Work out the finished part from the listing and answer in its coordinate system (mm). Face numbers are marked on the shaded views. A direction names the side the tool comes from. Round coordinates to 2 decimals unless told otherwise and drop trailing zeros. Loops run counter-clockwise (first coordinate to the right, second up) from the corner with the lowest first, then second, coordinate; pieces in that order, holes last.
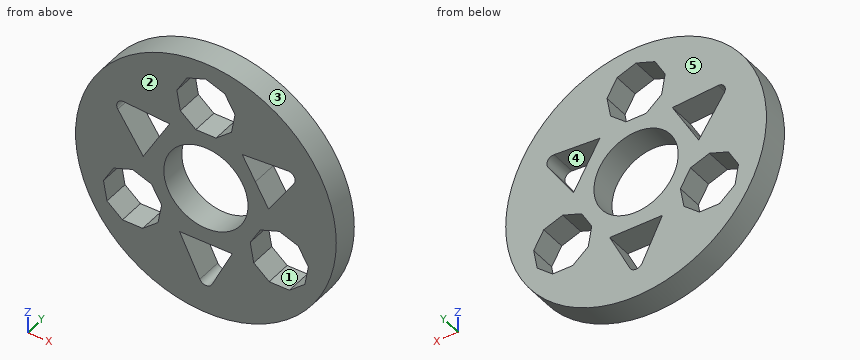
```python
from build123d import *

# Parameters (mm, degrees)
F0_R     = 24.75
F0_R_2   = 8
F1_DEPTH = 2.5
F3_DEPTH = 5.001


with BuildPart() as f1:
    # F0 (on Front) → F1 (new body, symmetric)
    with BuildSketch(Plane.XZ):
        Circle(F0_R)
        Circle(F0_R_2, mode=Mode.SUBTRACT)
    extrude(amount=F1_DEPTH, both=True)

    # F2 (on face) → F3 (cut, through all)
    with BuildSketch(Plane.XZ.offset(2.5)):
        Polygon((-1.916116, 10.819963), (1.916116, 10.819963), (4.851777, 13.283275), (5.517237, 17.057287), (3.601121, 20.376098), (0, 21.686799), (-3.601121, 20.376098), (-5.517237, 17.057287), (-4.851777, 13.283275), align=None)
        Polygon((-19.446779, -7.069387), (-18.781318, -10.843399), (-15.845658, -13.306711), (-12.013425, -13.306711), (-9.077765, -10.843399), (-8.412305, -7.069387), (-10.328421, -3.750576), (-13.929542, -2.439876), (-17.530662, -3.750576), align=None)
        Polygon((15.845658, -13.306711), (18.781318, -10.843399), (19.446779, -7.069387), (17.530662, -3.750576), (13.929542, -2.439876), (10.328421, -3.750576), (8.412305, -7.069387), (9.077765, -10.843399), (12.013425, -13.306711), align=None)
        with BuildLine():
            ThreePointArc((-1.158459, -18.64352), (0, -19.363865), (1.158459, -18.64352))
            Line((1.158459, -18.64352), (5.005436, -10.843399))
            Line((5.005436, -10.843399), (0, -10.843399))
            Line((0, -10.843399), (-5.005436, -10.843399))
            Line((-5.005436, -10.843399), (-1.158459, -18.64352))
        make_face()
        with BuildLine():
            Line((9.390659, 5.4217), (11.893377, 1.086865))
            Line((11.893377, 1.086865), (16.724992, 8.318505))
            ThreePointArc((16.724992, 8.318505), (16.769599, 9.681932), (15.566532, 10.325015))
            Line((15.566532, 10.325015), (6.887941, 9.756534))
            Line((6.887941, 9.756534), (9.390659, 5.4217))
        make_face()
        with BuildLine():
            Line((-9.390659, 5.4217), (-6.887941, 9.756534))
            Line((-6.887941, 9.756534), (-15.566532, 10.325015))
            ThreePointArc((-15.566532, 10.325015), (-16.769599, 9.681932), (-16.724992, 8.318505))
            Line((-16.724992, 8.318505), (-11.893377, 1.086865))
            Line((-11.893377, 1.086865), (-9.390659, 5.4217))
        make_face()
    extrude(amount=-F3_DEPTH, mode=Mode.SUBTRACT)


solid = f1.part
```
1. Given pin 1 (1.1 mm diameter, centred on x = 13.5, y = -1, fed in from +Z); pin 2 (1 mm diameter, centred on y = -1.5, z = -3, fed in from -X); pin 3 (1.5 mm diameter, centred on x = 15.5, y = 0, fed in from +Z), each flat-ended and moving along its own axis, determine where each tip first touches the part or whether it passes through.
Answer key:
pin 1: stops at z = 21.09
pin 2: stops at x = -24.62
pin 3: stops at z = 19.87
2. Consider probe 1 along Z at (x, y) = (0, -0.4); probe 2 along X at (y, z) = (0.35, -4.5); probe 3 along X at (y, z) = (-1.2, -13). Determine where each line is inside the solid, lowest interval first.
Answer key:
probe 1: z = -24.75 to -19.36, -10.84 to -8, 8 to 10.82, 21.69 to 24.75
probe 2: x = -24.34 to -17.96, -9.9 to -6.61, 6.61 to 9.9, 17.96 to 24.34
probe 3: x = -21.06 to -16.21, -11.65 to -3.94, 3.94 to 11.65, 16.21 to 21.06
3. Which of the six approach directions +Z, -Z, +X, -X, +Y, -Y give full straight-line access (tool end or side, diameter ignored) to the marked faces 1 and 2?
Answer key:
face 1: +Y, -Y
face 2: +Z, -Z, +X, -X, -Y
4. Determine the mould class of the marked faces 3, 4 and 5 for opening direction Z: +Z half, -Z half, draft (parallel to the pull), parting line (faces both ways), or undercut.
Answer key:
face 3: parting line
face 4: undercut
face 5: draft
5. Find section B-B (z = 9). Write down the section's boundary in (x, y), then the cut area to 3 significant figures.
Answer key:
outline: (-23.06, -2.5) - (-16.94, -2.5) - (-16.94, 2.5) - (-23.06, 2.5) - close; (-7.32, -2.5) - (7.32, -2.5) - (7.32, 2.5) - (-7.32, 2.5) - close; (16.94, -2.5) - (23.06, -2.5) - (23.06, 2.5) - (16.94, 2.5) - close
area: 134 mm2
6. Find section C-C (y = -0.45). Give the number of separate pieces and of enclosed holes in the cut face, then the cut area to 3 significant figures.
Answer key:
separate pieces: 1
enclosed holes: 7
area: 1,300 mm2
7. Find section A-A (z = 0). Write down the section's boundary in (x, y), then the cut area to 4 significant figures.
Answer key:
outline: (-24.75, -2.5) - (-8, -2.5) - (-8, 2.5) - (-24.75, 2.5) - close; (8, -2.5) - (24.75, -2.5) - (24.75, 2.5) - (8, 2.5) - close
area: 167.5 mm2
